Work out the finished part from the listing and answer in its coordinate system (mm). Face numbers are marked on the shaded views. A direction names the side the tool comes from. Coordinates: 2 decimals unless noted, no trailing zeros. Loops run counter-clockwise (first coordinate to the right, second up) from the corner with the lowest first, then second, coordinate; pieces in that order, holes last. Notation, with made-up numbers: (40.25, 20.5) -> (68.25, 20.5) arc R15 cw to (68.25, 28.5) -> close; hole circle Ø4 at (-38.75, 15). An arc over 180 degrees is marked (long way). Answer as CSV lines item,"result".
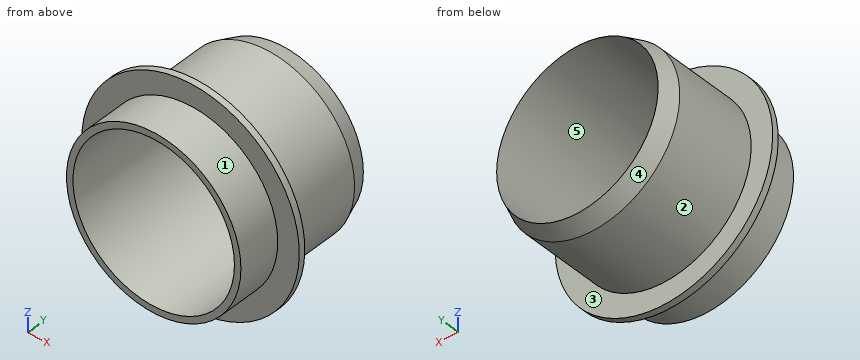
```python
from build123d import *

# Parameters (mm, degrees)
SKETCH_1_R        = 40.5
SKETCH_1_R_2      = 37.5
EXTRUDE_1_DEPTH   = 70
SKETCH_3_R        = 50.5
SKETCH_3_R_2      = 40.5
EXTRUDE_1_2_DEPTH = 3


# Read off the part's stored shape, not the designer's step: Вырез-Повернуть-Тонкостенный1
with BuildPart() as part:
    # Эскиз1 → Extrude 1 (new body)
    with BuildSketch(Plane(origin=(0, 0, 0), x_dir=(1, 0, 0), z_dir=(0, 1, 0))):
        Circle(SKETCH_1_R)
        Circle(SKETCH_1_R_2, mode=Mode.SUBTRACT)
    extrude(amount=EXTRUDE_1_DEPTH)

    # Вырез-Повернуть-Тонкостенный1 outline → Вырез-Повернуть-Тонкостенный1 (revolve, cut)
    with BuildSketch(Plane.XY):
        Polygon((40.5, 70), (37.5, 70), (40.5, 61.757567742), align=None)
    revolve(axis=Axis((0, 0, 0), (0, 1, 0)), mode=Mode.SUBTRACT)

    # Эскиз3 → Extrude 1 2 (add)
    with BuildSketch(Plane(origin=(0, 20, 0), x_dir=(1, 0, 0), z_dir=(0, 1, 0))):
        with Locations(Location((0, 0, 0), (0, 0, 270))):
            Circle(SKETCH_3_R)
        Circle(SKETCH_3_R_2, mode=Mode.SUBTRACT)
    extrude(amount=EXTRUDE_1_2_DEPTH)


solid = part.part
```
(1) Flat-ended cylindrical pins translate along their axes: pin 1 Ø8 at (y, z) = (46.5, 24.5) entering from +X; pin 2 Ø1 at (x, z) = (-37, -32) entering from +Y; pin 3 Ø12 at (x, y) = (-38.5, 20.5) entering from -Z; pin 4 Ø2 at (x, z) = (-10, 34) entering from -Y. Find the tip coordinate at first contact, or state that the pin passes through.
Computed values:
pin 1,"x = 34.93"
pin 2,"y = 23"
pin 3,"z = -38.65"
pin 4,"through"
(2) A cutting plane is placed at A-A, the plane z = 0. Write down the section's boundary in (x, y).
Computed values:
outline,"(-50.5, 20) -> (-40.5, 20) -> (-40.5, 0) -> (-37.5, 0) -> (-37.5, 70) -> (-40.5, 61.76) -> (-40.5, 23) -> (-50.5, 23) -> close; (37.5, 0) -> (40.5, 0) -> (40.5, 20) -> (50.5, 20) -> (50.5, 23) -> (40.5, 23) -> (40.5, 61.76) -> (37.5, 70) -> close"
(3) A cutting plane is placed at B-B, the plane x = 0. Write down the section's boundary in (y, z).
Computed values:
outline,"(0, -40.5) -> (20, -40.5) -> (20, -50.5) -> (23, -50.5) -> (23, -40.5) -> (61.76, -40.5) -> (70, -37.5) -> (0, -37.5) -> close; (0, 37.5) -> (70, 37.5) -> (61.76, 40.5) -> (23, 40.5) -> (23, 50.5) -> (20, 50.5) -> (20, 40.5) -> (0, 40.5) -> close"
(4) A cutting plane is placed at D-D, the plane x = -42. Write down the section's boundary in (y, z), and give its area (3 significant figures).
Computed values:
outline,"(20, -28.04) -> (23, -28.04) -> (23, 28.04) -> (20, 28.04) -> close"
area,"168 mm2"
(5) Consider line 1 along Z through (x, y) = (0, 34); line 2 along X through (y, z) = (26, -24). Determine where each line is inside the solid, lowest interval first.
Computed values:
line 1,"-40.5 to -37.5, 37.5 to 40.5"
line 2,"-32.62 to -28.81, 28.81 to 32.62"
(6) A cutting plane is placed at C-C, the plane y = 17. Write down the section's boundary in (x, z).
Computed values:
outline,"circle Ø81 at (0, 0); hole circle Ø75 at (0, 0)"
(7) Which of the six approach directions +Z, -Z, +X, -X, +Y, -Y give full straight-line access (tool end or side, diameter ignored) to the marked faces 1 and 2?
Computed values:
face 1,"-Y"
face 2,"+Y"
(8) For a pull along X with two mould halves and no side action, classify the marked faces 3, 4 and 5 as pulls with the +X half, pulls with the -X half, needs draft (parallel to the pull), parting line crosses it, or undercut.
Computed values:
face 3,"needs draft"
face 4,"parting line crosses it"
face 5,"undercut"
